Could you check a few things on this drawing? It's one solid part, dimensions in mm from its lowest x, y, z. Give positions to 0.01 mm unless a question says otherwise; leave off trailing zeros. Write each loop counter-clockwise with the first axis right and the second up, starting at its lowest first coordinate (ties: lowest second). Pieces come first, ordered by that corner, then holes. Notation, with made-up numbers: M -39.75,65 L 1.25,65 A12 ccw 1.25,78 Z; hole C -29.75,-22 d6. An arc over 180 degrees is marked long. Write each question's results on one line, items separated by ' | '. Start each with the question number.
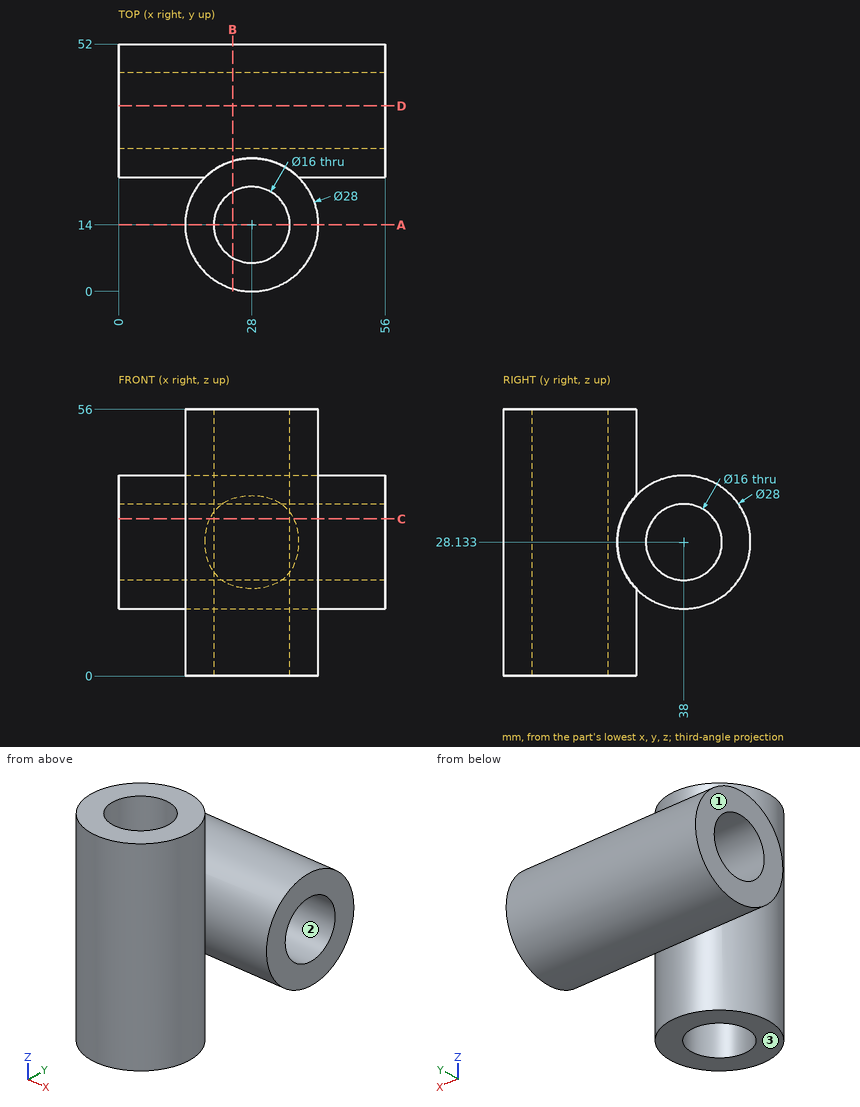
Q1. If we section it at D-D (y = 39): Please give me the cut outline in (x, z) (1 decimal), plus the area to 3 significant figures.
Q2. If we section it at C-C (z = 33): Please give me the cut outline in (x, y), plus the area to 3 significant figures.
Q3. If we section it at A-A (y = 14): Please give me the cut outline in (x, z), plus the area to 3 significant figures.
Q4. Please list where these lines run through material, in increasing order: line 1 (Y direction, x = 27.5, z = 45) (1 decimal); line 2 (Y direction, x = 28, z = 35) (1 decimal); line 3 (Y direction, x = 29.5, z = 49). Write a range as [from, to].
Q5. If we mould it in two halves opening along Z, with no side actions, what happens to the marked faces 1, 2 and 3? For each: pulls with the +Z half, pulls with the -Z half, needs draft (parallel to the pull), parting line crosses it, or undercut.
Q6. I'm going to push flat-ended pins straight in: P1, Ø12, axis at y = 31, z = 8, coming from the -X side; P2, Ø2, axis at x = 15.5, z = 47, coming from the +Y side (1 decimal); P3, Ø4, axis at x = 49, y = 39.5, coming from the -Z side. Where does each tip first touch, or does it pass through?
Q7. If we section it at B-B (x = 24): Please give me the cut outline in (y, z).
Determined:
1) outline: M 0,14.2 L 56,14.2 L 56,20.2 L 0,20.2 Z; M 0,36.1 L 56,36.1 L 56,42.1 L 0,42.1 Z | area: 675 mm²
2) outline: M 0,24.87 L 19.18,24.87 A14 ccw long 36.82,24.87 L 56,24.87 L 56,31.65 L 0,31.65 Z; M 0,44.35 L 56,44.35 L 56,51.13 L 0,51.13 Z; hole C 28,14 d16 | area: 1,140 mm²
3) outline: M 14,0 L 20,0 L 20,56 L 14,56 Z; M 36,0 L 42,0 L 42,56 L 36,56 Z | area: 672 mm²
4) line 1: y = [0, 6], [22, 28] | line 2: y = [0, 6], [22, 33.9], [42.1, 50.2] | line 3: y = [0.08, 6.14], [21.86, 27.92]
5) face 1: needs draft | face 2: undercut | face 3: pulls with the -Z half
6) P1: stops at x = 19.34 | P2: stops at y = 22 | P3: stops at z = 14.13
7) outline: M 0.58,0 L 7.07,0 L 7.07,56 L 0.58,56 Z; M 20.93,0 L 27.42,0 L 27.42,18.97 A14 ccw long 27.42,37.3 L 27.42,56 L 20.93,56 Z; hole C 38,28.13 d16
